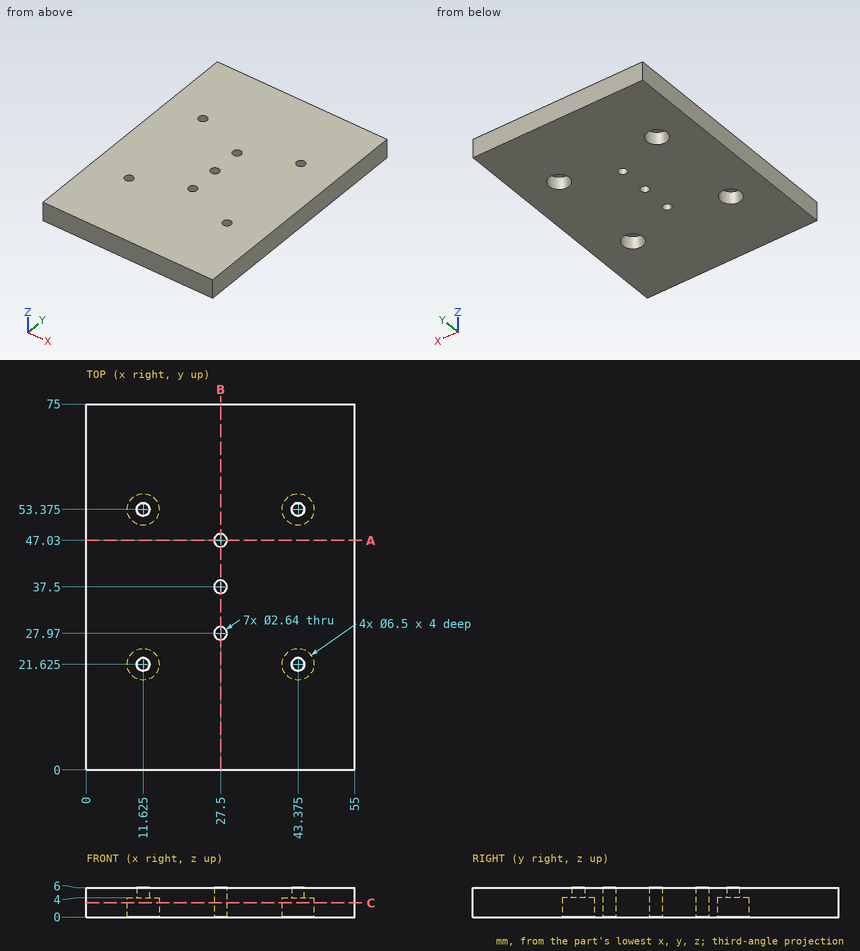
Geometry check sheet. Reference: drawing and pictorial views, mm from the part's lowest x, y, z. Coordinates: 2 decimals unless noted, no trailing zeros. Order: outer loops, then holes, each group sorted by start corner. A loop starts at its lowest first (then second) coordinate and runs counter-clockwise, first axis right, second up. Notation, with made-up numbers: M 26,-20 L 65,-20 A21 cw 65,-14 Z; hole C -18,49.25 d2. An arc over 180 degrees is marked long. Write each question's results on one line, items separated by ' | '. Start each with the question number.
1. Material ranges on probe 1 along Y at (x, z) = (14, 2.3); probe 2 along X at (y, z) = (47, 3.25); probe 3 along Y at (x, z) = (28.5, 3.2), recorded low to high.
2. Cross-section at C-C on z = 2.9. Record the cut outline in (x, y) (3 decimals), and give its area (3 significant figures).
3. Cross-section at A-A on y = 47.03. Record the cut outline in (x, z), and give its area (3 significant figures).
4. Cross-section at B-B on x = 27.5. Record the cut outline in (y, z).
5. Go/stop test with flat-tipped pins: P1, Ø3, axis at x = 43.5, y = 22, coming from the -Z side; P2, Ø2.5, axis at x = 43.375, y = 53.375, coming from the -Z side. Record where each tip stops, or that it passes through.
Checks:
1) probe 1: y = 0 to 19.41, 23.84 to 51.16, 55.59 to 75 | probe 2: x = 0 to 26.18, 28.82 to 55 | probe 3: y = 0 to 27.11, 28.83 to 36.64, 38.36 to 46.17, 47.89 to 75
2) outline: M 0,0 L 55,0 L 55,75 L 0,75 Z; hole C 11.625,21.625 d6.5; hole C 11.625,53.375 d6.5; hole C 27.5,27.97 d2.64; hole C 27.5,37.5 d2.64; hole C 27.5,47.03 d2.64; hole C 43.375,21.625 d6.5; hole C 43.375,53.375 d6.5 | area: 3,980 mm²
3) outline: M 0,0 L 26.18,0 L 26.18,6 L 0,6 Z; M 28.82,0 L 55,0 L 55,6 L 28.82,6 Z | area: 314 mm²
4) outline: M 0,0 L 26.65,0 L 26.65,6 L 0,6 Z; M 29.29,0 L 36.18,0 L 36.18,6 L 29.29,6 Z; M 38.82,0 L 45.71,0 L 45.71,6 L 38.82,6 Z; M 48.35,0 L 75,0 L 75,6 L 48.35,6 Z
5) P1: stops at z = 4 | P2: passes through
